```python
from build123d import *

# Parameters (mm, degrees)
SKETCH1_W           = 69.85
SKETCH1_H           = 69.85
BOSS_EXTRUDE1_DEPTH = 4
SKETCH2_R           = 11.90625
BOSS_EXTRUDE2_DEPTH = 5
SKETCH3_R           = 1.7859375
CUT_EXTRUDE1_DEPTH  = 9


with BuildPart() as part:
    # Sketch1 → Boss-Extrude1 (new body)
    with BuildSketch(Plane(origin=(0, 0, 0), x_dir=(1, 0, 0), z_dir=(0, 1, 0))):
        with Locations((34.925, 34.925)):
            Rectangle(SKETCH1_W, SKETCH1_H)
    extrude(amount=BOSS_EXTRUDE1_DEPTH)

    # Sketch2 → Boss-Extrude2 (add)
    with BuildSketch(Plane(origin=(0, 4, 0), x_dir=(1, 0, 0), z_dir=(0, 1, 0))):
        with Locations((34.925, 34.925)):
            Circle(SKETCH2_R)
    extrude(amount=BOSS_EXTRUDE2_DEPTH)

    # Sketch3 → Cut-Extrude1 (cut)
    with BuildSketch(Plane(origin=(0, 9, 0), x_dir=(1, 0, 0), z_dir=(0, 1, 0))):
        with Locations((29.9640625, 34.925)):
            Circle(SKETCH3_R)
        with Locations((39.8859375, 34.925)):
            Circle(SKETCH3_R)
    extrude(amount=-CUT_EXTRUDE1_DEPTH, mode=Mode.SUBTRACT)


solid = part.part
```
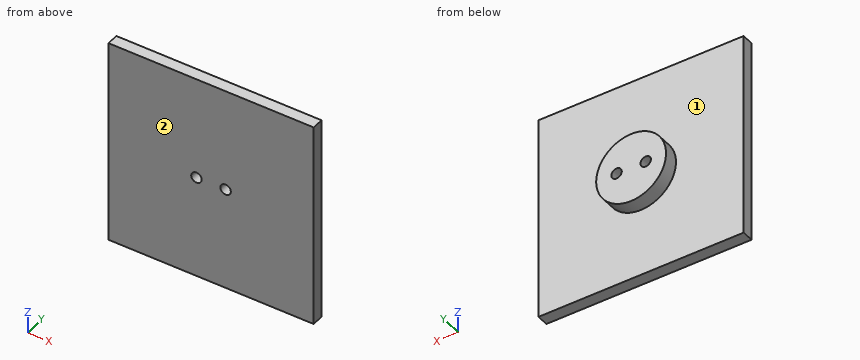
Check sheet for the modelled part. Datum: model origin and axes. Units: mm. Face numbers are marked on the shaded views. Give positions to 0.01 mm unless a question says otherwise; leave off trailing zeros. Loops run counter-clockwise (first coordinate to the right, second up) from the corner with the lowest first, then second, coordinate; pieces in that order, holes last. Notation, with made-up numbers: M -15.5,20.5 L 15.5,20.5 A15 cw 15.5,27.5 Z; hole C 9.25,-28.75 d7. An arc over 180 degrees is marked long. Answer as CSV lines item,"result".
Item 1: Sectioned sample at A-A, the plane z = -27.5. Enter the section's corners in (x, y).
Reply:
outline,"M 0,0 L 69.85,0 L 69.85,4 L 44.23,4 L 44.23,9 L 25.62,9 L 25.62,4 L 0,4 Z"
Item 2: Sectioned sample at D-D, the plane x = 60. Enter the section's corners in (y, z).
Reply:
outline,"M 0,-69.85 L 4,-69.85 L 4,0 L 0,0 Z"
Item 3: Sectioned sample at C-C, the plane y = 5.5. State how many separate pieces and enclosed holes the cut face has, then the cut area to 3 significant figures.
Reply:
separate pieces,"1"
enclosed holes,"2"
area,"425 mm^2"
Item 4: Depth check by flat-ended pin: pin 1 Ø2 at (x, y) = (25.5, 8) entering from -Z; pin 2 Ø12 at (x, z) = (62.5, -15) entering from +Y. Enter the tip coordinate at first touch or a pass-through.
Reply:
pin 1,"z = -43.34"
pin 2,"y = 4"
Item 5: Scan lines: L1, parallel to Y at x = 10.5, z = -60; L2, parallel to Z at x = 37, y = 7.5; L3, parallel to X at y = 8.5, z = -27.5. Record each from-to range of solid material in increasing order.
Reply:
L1,"0 to 4"
L2,"-46.65 to -23.2"
L3,"25.62 to 44.23"
Item 6: Draft check along Y on the marked faces 1 and 2. Enter one of: pulls with the +Y half, pulls with the -Y half, needs draft (parallel to the pull), parting line crosses it, or undercut.
Reply:
face 1,"pulls with the +Y half"
face 2,"pulls with the -Y half"
Item 7: Sectioned sample at B-B, the plane x = 27. Enter the section's corners in (y, z), then the cut area to 3 significant figures.
Reply:
outline,"M 0,-69.85 L 4,-69.85 L 4,-43.81 L 9,-43.81 L 9,-26.04 L 4,-26.04 L 4,0 L 0,0 Z"
area,"368 mm^2"
